from build123d import *

# Parameters (mm, degrees)
CROQUIS1_W                          = 90
CROQUIS1_H                          = 50
SALIENTE_EXTRUIR1_DEPTH             = 5
CROQUIS4_W                          = 90
CROQUIS4_H                          = 5
SALIENTE_EXTRUIR2_DEPTH             = 49.5
CROQUIS5_W                          = 60
CROQUIS5_H                          = 5
SALIENTE_EXTRUIR3_DEPTH             = 35
CROQUIS11_W                         = 75
CROQUIS11_H                         = 80
CORTAR_EXTRUIR3_DEPTH               = 2.5
SALIENTE_EXTRUIR4_REACH             = 27
SALIENTE_EXTRUIR4_DIRECTION_2_REACH = 26.5
CROQUIS13_W                         = 90
CROQUIS13_H                         = 5
CORTAR_EXTRUIR4_DEPTH               = 1
CROQUIS15_W                         = 54
CROQUIS15_H                         = 3
SALIENTE_EXTRUIR5_DEPTH             = 50
CROQUIS18_W                         = 90
CROQUIS18_H                         = 5
CORTAR_EXTRUIR5_DEPTH               = 1
SALIENTE_EXTRUIR6_REACH             = 47
SALIENTE_EXTRUIR6_DIRECTION_2_REACH = 47
SALIENTE_EXTRUIR7_DEPTH             = 20
CROQUIS24_W                         = 20
CROQUIS24_H                         = 15
SALIENTE_EXTRUIR8_DEPTH             = 54
CROQUIS25_W                         = 15.6
CROQUIS25_H                         = 12.6
CORTAR_EXTRUIR6_DEPTH               = 54
CROQUIS26_W                         = 39
CROQUIS26_H                         = 15
CORTAR_EXTRUIR7_DEPTH               = 20


with BuildPart() as part:
    # Croquis1 → Saliente-Extruir1 (new body)
    with BuildSketch(Plane(origin=(0, 0, 0), x_dir=(1, 0, 0), z_dir=(0, 1, 0))):
        Rectangle(CROQUIS1_W, CROQUIS1_H)
    extrude(amount=SALIENTE_EXTRUIR1_DEPTH)

    # Croquis4 → Saliente-Extruir2 (add)
    with BuildSketch(Plane(origin=(0, 5, 0), x_dir=(1, 0, 0), z_dir=(0, 1, 0))):
        with Locations((0, 27.5)):
            Rectangle(CROQUIS4_W, CROQUIS4_H)
    extrude(amount=-SALIENTE_EXTRUIR2_DEPTH)

    # Croquis5 → Saliente-Extruir3 (add)
    with BuildSketch(Plane(origin=(0, 0, -30), x_dir=(-1, 0, 0), z_dir=(0, 0, -1))):
        with Locations((0, -22)):
            Rectangle(CROQUIS5_W, CROQUIS5_H)
    extrude(amount=SALIENTE_EXTRUIR3_DEPTH)

    # Croquis11 → Cortar-Extruir3 (cut)
    with BuildSketch(Plane(origin=(0, 5, 0), x_dir=(1, 0, 0), z_dir=(0, 1, 0))):
        with Locations((0, 18)):
            Rectangle(CROQUIS11_W, CROQUIS11_H)
    extrude(amount=-CORTAR_EXTRUIR3_DEPTH, mode=Mode.SUBTRACT)

    # Saliente-Extruir4: up to this face of the body (flat: up to its plane)
    saliente_extruir4_end = Plane(part.part.faces().sort_by_distance((0, -44.5, -27.5))[0])
    # Croquis12 → Saliente-Extruir4 (add, up to the picked face)
    with BuildSketch(Plane(origin=(0, -19.5, 0), x_dir=(1, 0, 0), z_dir=(0, 1, 0)), mode=Mode.PRIVATE) as saliente_extruir4_sk1:
        Polygon((-39.591673087, 75), (-45, 75), (-30, 65), (30, 65), (45, 75), (39.591673087, 75), (29.091673087, 68), (28.908326913, 68), (26.008326913, 70), (23.108326913, 68), (20.208326913, 70), (17.308326913, 68), (14.408326913, 70), (11.508326913, 68), (8.608326913, 70), (5.708326913, 68), (2.808326913, 70), (-0.091673087, 68), (-2.991673087, 70), (-5.891673087, 68), (-8.791673087, 70), (-11.691673087, 68), (-14.591673087, 70), (-17.491673087, 68), (-20.391673087, 70), (-23.291673087, 68), (-26.191673087, 70), (-29.091673087, 68), align=None)
    saliente_extruir4_tool1 = split(extrude(saliente_extruir4_sk1.sketch, amount=-SALIENTE_EXTRUIR4_REACH, mode=Mode.PRIVATE), bisect_by=saliente_extruir4_end, keep=Keep.BOTH, mode=Mode.PRIVATE)
    add(saliente_extruir4_tool1.solids().sort_by_distance((-27.127569, -19.5, -68.254549))[0])

    # Saliente-Extruir4 direction 2: up to this face of the body (flat: up to its plane)
    saliente_extruir4_direction_2_end = Plane(part.part.faces().sort_by_distance((0, 2.5, -4))[0])
    # Croquis12 → Saliente-Extruir4 direction 2 (add, up to the picked face)
    with BuildSketch(Plane(origin=(0, -19.5, 0), x_dir=(1, 0, 0), z_dir=(0, 1, 0)), mode=Mode.PRIVATE) as saliente_extruir4_direction_2_sk1:
        Polygon((-39.591673087, 75), (-45, 75), (-30, 65), (30, 65), (45, 75), (39.591673087, 75), (29.091673087, 68), (28.908326913, 68), (26.008326913, 70), (23.108326913, 68), (20.208326913, 70), (17.308326913, 68), (14.408326913, 70), (11.508326913, 68), (8.608326913, 70), (5.708326913, 68), (2.808326913, 70), (-0.091673087, 68), (-2.991673087, 70), (-5.891673087, 68), (-8.791673087, 70), (-11.691673087, 68), (-14.591673087, 70), (-17.491673087, 68), (-20.391673087, 70), (-23.291673087, 68), (-26.191673087, 70), (-29.091673087, 68), align=None)
    saliente_extruir4_direction_2_tool1 = split(extrude(saliente_extruir4_direction_2_sk1.sketch, amount=SALIENTE_EXTRUIR4_DIRECTION_2_REACH, mode=Mode.PRIVATE), bisect_by=saliente_extruir4_direction_2_end, keep=Keep.BOTH, mode=Mode.PRIVATE)
    add(saliente_extruir4_direction_2_tool1.solids().sort_by_distance((-27.127569, -19.5, -68.254549))[0])

    # Croquis13 → Cortar-Extruir4 (cut)
    with BuildSketch(Plane.XZ.offset(44.5)):
        with Locations((0, -27.5)):
            Rectangle(CROQUIS13_W, CROQUIS13_H)
        Polygon((-39.591673087, -75), (-29.091673087, -68), (-26.191673087, -70), (-23.291673087, -68), (-20.391673087, -70), (-17.491673087, -68), (-14.591673087, -70), (-11.691673087, -68), (-8.791673087, -70), (-5.891673087, -68), (-2.991673087, -70), (-0.091673087, -68), (2.808326913, -70), (5.708326913, -68), (8.608326913, -70), (11.508326913, -68), (14.408326913, -70), (17.308326913, -68), (20.208326913, -70), (23.108326913, -68), (26.008326913, -70), (28.908326913, -68), (29.091673087, -68), (39.591673087, -75), (45, -75), (30, -65), (-30, -65), (-45, -75), align=None)
    extrude(amount=-CORTAR_EXTRUIR4_DEPTH, mode=Mode.SUBTRACT)

    # Croquis15 → Saliente-Extruir5 (add)
    with BuildSketch(Plane.XY.offset(-25)):
        with Locations((0, -39.25)):
            Rectangle(CROQUIS15_W, CROQUIS15_H)
    extrude(amount=SALIENTE_EXTRUIR5_DEPTH)

    # Croquis18 → Cortar-Extruir5 (cut)
    with BuildSketch(Plane.XZ.offset(43.5)):
        with Locations((0, -27.5)):
            Rectangle(CROQUIS18_W, CROQUIS18_H)
        Polygon((-45, -75), (-39.591673087, -75), (-29.091673087, -68), (-26.191673087, -70), (-23.291673087, -68), (-20.391673087, -70), (-17.491673087, -68), (-14.591673087, -70), (-11.691673087, -68), (-8.791673087, -70), (-5.891673087, -68), (-2.991673087, -70), (-0.091673087, -68), (2.808326913, -70), (5.708326913, -68), (8.608326913, -70), (11.508326913, -68), (14.408326913, -70), (17.308326913, -68), (20.208326913, -70), (23.108326913, -68), (26.008326913, -70), (28.908326913, -68), (29.091673087, -68), (39.591673087, -75), (45, -75), (30, -65), (-30, -65), align=None)
    extrude(amount=-CORTAR_EXTRUIR5_DEPTH, mode=Mode.SUBTRACT)

    # Saliente-Extruir6: up to this face of the body (flat: up to its plane)
    saliente_extruir6_end = Plane(part.part.faces().sort_by_distance((-27, -39.25, 0))[0])
    # Croquis22 → Saliente-Extruir6 (add, up to the picked face)
    with BuildSketch(Plane(origin=(0, 0, 0), x_dir=(0, 0, -1), z_dir=(1, 0, 0)), mode=Mode.PRIVATE) as saliente_extruir6_sk1:
        Polygon((25, -37.75), (25, -32.75), (20, -37.75), align=None)
    saliente_extruir6_tool1 = split(extrude(saliente_extruir6_sk1.sketch, amount=-SALIENTE_EXTRUIR6_REACH, mode=Mode.PRIVATE), bisect_by=saliente_extruir6_end, keep=Keep.BOTH, mode=Mode.PRIVATE)
    add(saliente_extruir6_tool1.solids().sort_by_distance((0, -36.083333, -23.333333))[0])

    # Saliente-Extruir6 direction 2: up to this face of the body (flat: up to its plane)
    saliente_extruir6_direction_2_end = Plane(part.part.faces().sort_by_distance((27, -39.25, 0))[0])
    # Croquis22 → Saliente-Extruir6 direction 2 (add, up to the picked face)
    with BuildSketch(Plane(origin=(0, 0, 0), x_dir=(0, 0, -1), z_dir=(1, 0, 0)), mode=Mode.PRIVATE) as saliente_extruir6_direction_2_sk1:
        Polygon((25, -37.75), (25, -32.75), (20, -37.75), align=None)
    saliente_extruir6_direction_2_tool1 = split(extrude(saliente_extruir6_direction_2_sk1.sketch, amount=SALIENTE_EXTRUIR6_DIRECTION_2_REACH, mode=Mode.PRIVATE), bisect_by=saliente_extruir6_direction_2_end, keep=Keep.BOTH, mode=Mode.PRIVATE)
    add(saliente_extruir6_direction_2_tool1.solids().sort_by_distance((0, -36.083333, -23.333333))[0])

    # Croquis23 → Saliente-Extruir7 (add, symmetric)
    with BuildSketch(Plane(origin=(0, 0, 0), x_dir=(0, 0, -1), z_dir=(1, 0, 0))):
        Polygon((38.45, -4.5), (56.55, -4.5), (56.55, -19.5), (59.55, -19.5), (59.55, -1.5), (35.45, -1.5), (35.45, -19.5), (38.45, -19.5), align=None)
    extrude(amount=SALIENTE_EXTRUIR7_DEPTH, both=True)

    # Croquis24 → Saliente-Extruir8 (add)
    with BuildSketch(Plane.ZY.offset(27)):
        with Locations((10, -30.25)):
            Rectangle(CROQUIS24_W, CROQUIS24_H)
    extrude(amount=-SALIENTE_EXTRUIR8_DEPTH)

    # Croquis25 → Cortar-Extruir6 (cut)
    with BuildSketch(Plane.ZY.offset(27)):
        with Locations((10, -31.45)):
            Rectangle(CROQUIS25_W, CROQUIS25_H)
    extrude(amount=-CORTAR_EXTRUIR6_DEPTH, mode=Mode.SUBTRACT)

    # Croquis26 → Cortar-Extruir7 (cut)
    with BuildSketch(Plane.XY.offset(20)):
        with Locations((0, -30.25)):
            Rectangle(CROQUIS26_W, CROQUIS26_H)
    extrude(amount=-CORTAR_EXTRUIR7_DEPTH, mode=Mode.SUBTRACT)


solid = part.part
Read the model definition and answer for the solid it produces. Units are mm, in the model's axes. A direction names the side the tool comes from. Round coordinates to 2 decimals unless told otherwise and drop trailing zeros. Loops run counter-clockwise (first coordinate to the right, second up) from the corner with the lowest first, then second, coordinate; pieces in that order, holes last. Notation, with made-up numbers: (14.5, 58) - (36.5, 58) arc R23 cw to (36.5, 73) - close; hole circle Ø6 at (-15.5, 89.5). An arc over 180 degrees is marked (long way). One line per question, with ' | ' between items. Start each with the question number.
Q1. Flat-ended cylindrical pins translate along their axes: pin 1 (8 mm diameter, centred on x = 23, z = 11, fed in from -Y); pin 2 (5.5 mm diameter, centred on y = -30, z = 1.5, fed in from -X); pin 3 (5 mm diameter, centred on x = -18.5, z = -72, fed in from +Y); pin 4 (3 mm diameter, centred on x = -11.5, z = -61, fed in from -Y). Find the tip coordinate at first contact, or state that the pin passes through.
Q2. Section A-A on z = 7 is taken. Give the vertices of the cut face in (x, y).
Q3. For faces 1 (the flat face through (-37.605, -20.315, -70.07)), 2 (the flat face through (0, -12, -56.55)), 3 (the flat face through (0, -24.5, -47)), 4 (the flat face through (-23, -22.75, 10)), 5 (the flat face through (-16.021, -20.315, -69.014)), determine the directions among +Z, -Z, +X, -X, +Y, -Y from which every point of the face is accessible in a straight line to the end or side of a thin tool.
Q4. For a pull along Z with two mould halves and no side action, classify faces 6 (the flat face through (0, -10, -35.45)), 7 (the flat face through (37.395, -20.315, -69.93)), 8 (the flat face through (24.579, -20.315, -69.014)), 9 (the flat face through (-1, 0, 0)) as +Z half, -Z half, draft (parallel to the pull), parting line (faces both ways), or undercut.
Q5. Section B-B on z = -49.5 is taken. Give the vertices of the cut face in (x, y).
Q6. Find the intervals of material crossed by L1, parallel to Y at x = 13, z = -41.5; L2, parallel to Y at x = -11.5, z = -14; L3, parallel to X at y = 3.5, z = -29.5, in increasing order.
Q7. Section D-D on y = -6.5 is taken. Count the separate pieces of the cut face and the enclosed holes in it, plus the area to 3 significant figures.
Established:
1) pin 1: y = -40.75 | pin 2: x = -27 | pin 3: through | pin 4: y = -24.5
2) outline: (-45, 0) - (45, 0) - (45, 5) - (37.5, 5) - (37.5, 2.5) - (-37.5, 2.5) - (-37.5, 5) - (-45, 5) - close; (-27, -40.75) - (27, -40.75) - (27, -37.75) - (-27, -37.75) - close; (-27, -25.15) - (-19.5, -25.15) - (-19.5, -22.75) - (-27, -22.75) - close; (19.5, -25.15) - (27, -25.15) - (27, -22.75) - (19.5, -22.75) - close
3) face 1: -X, +Y, -Y | face 2: +X, -X | face 3: +X, -X, -Y | face 4: +Z, +X, -X | face 5: -Z, +Y, -Y
4) face 6: undercut | face 7: undercut | face 8: -Z half | face 9: draft
5) outline: (-30, -24.5) - (30, -24.5) - (30, -19.5) - (-30, -19.5) - close; (-20, -4.5) - (20, -4.5) - (20, -1.5) - (-20, -1.5) - close
6) L1: -24.5 to -19.5, -4.5 to -1.5 | L2: -40.75 to -37.75, 0 to 2.5 | L3: -45 to -37.5, 37.5 to 45
7) separate pieces: 4 | enclosed holes: 0 | area: 1,020 mm²
